```python
from build123d import *

# Parameters (mm, degrees)
SKETCH1_R                = 62.5
BOSS_EXTRUDE1_DEPTH      = 8
BOSS_EXTRUDE1_DEPTH_BACK = 8
SKETCH2_R                = 55
CUT_EXTRUDE1_DEPTH       = 5
SKETCH3_R                = 55
CUT_EXTRUDE2_DEPTH       = 5
SKETCH4_R                = 5
CUT_EXTRUDE3_DEPTH       = 12
SKETCH5_W                = 5
SKETCH5_H                = 25
CUT_EXTRUDE4_DEPTH       = 12
CIRPATTERN1_COUNT        = 4


with BuildPart() as part:
    # Sketch1 → Boss-Extrude1 (new body, two sides)
    with BuildSketch(Plane(origin=(0, 0, 0), x_dir=(1, 0, 0), z_dir=(0, 1, 0))) as boss_extrude1_sk:
        Circle(SKETCH1_R)
    extrude(amount=BOSS_EXTRUDE1_DEPTH)
    extrude(boss_extrude1_sk.sketch, amount=-BOSS_EXTRUDE1_DEPTH_BACK)

    # Sketch2 → Cut-Extrude1 (cut)
    with BuildSketch(Plane(origin=(0, 8, 0), x_dir=(1, 0, 0), z_dir=(0, 1, 0))):
        Circle(SKETCH2_R)
    extrude(amount=-CUT_EXTRUDE1_DEPTH, mode=Mode.SUBTRACT)

    # Sketch3 → Cut-Extrude2 (cut)
    with BuildSketch(Plane.XZ.offset(8)):
        Circle(SKETCH3_R)
    extrude(amount=-CUT_EXTRUDE2_DEPTH, mode=Mode.SUBTRACT)

    # Sketch4 → Cut-Extrude3 (cut, through all)
    with BuildSketch(Plane.XZ.offset(3)):
        Circle(SKETCH4_R)
    extrude(amount=-CUT_EXTRUDE3_DEPTH, mode=Mode.SUBTRACT)

    # Sketch5 → Cut-Extrude4 (cut, through all)
    with BuildSketch(Plane.XZ.offset(3)):
        with Locations((0, 40)):
            Rectangle(SKETCH5_W, SKETCH5_H)
    cut_extrude4 = extrude(amount=-CUT_EXTRUDE4_DEPTH, mode=Mode.SUBTRACT)

    # CirPattern1: Cut-Extrude4 ×4 about axis
    cirpattern1_axis = Axis((0, 0, 0), (0, 1, 0))
    for i in range(1, CIRPATTERN1_COUNT):
        add(cut_extrude4.rotate(cirpattern1_axis, i * 360 / CIRPATTERN1_COUNT), mode=Mode.SUBTRACT)


solid = part.part
```
Work out the finished part from the listing and answer in its coordinate system (mm). A direction names the side the tool comes from. Give positions to 0.01 mm unless a question says otherwise; leave off trailing zeros. Loops run counter-clockwise (first coordinate to the right, second up) from the corner with the lowest first, then second, coordinate; pieces in that order, holes last. Notation, with made-up numbers: (2, 47) -> (23, 47) arc R21 ccw to (23, 51) -> close; hole circle Ø4 at (-34, 39). An arc over 180 degrees is marked (long way). Use CSV: the item, a comma, the result in double quotes.
1. The part is cut by section D-D (z = 30). Write down the section's boundary in (x, y).
Found:
outline,"(-54.83, -8) -> (-46.1, -8) -> (-46.1, -3) -> (-2.5, -3) -> (-2.5, 3) -> (-46.1, 3) -> (-46.1, 8) -> (-54.83, 8) -> close; (2.5, -3) -> (46.1, -3) -> (46.1, -8) -> (54.83, -8) -> (54.83, 8) -> (46.1, 8) -> (46.1, 3) -> (2.5, 3) -> close"
2. Straight lines are drawn through the part: line 1 (Z direction, x = 0, y = 1.8); line 2 (Z direction, x = 0, y = 6.25); line 3 (Y direction, x = 4.5, z = 32.5). For each, find the intervals that lie inside material, in ascending order.
Found:
line 1,"-62.5 to -52.5, -27.5 to -5, 5 to 27.5, 52.5 to 62.5"
line 2,"-62.5 to -55, 55 to 62.5"
line 3,"-3 to 3"
3. The part is cut by section C-C (z = 0). Write down the section's boundary in (x, y).
Found:
outline,"(-62.5, -8) -> (-55, -8) -> (-55, -3) -> (-52.5, -3) -> (-52.5, 3) -> (-55, 3) -> (-55, 8) -> (-62.5, 8) -> close; (-27.5, -3) -> (-5, -3) -> (-5, 3) -> (-27.5, 3) -> close; (5, -3) -> (27.5, -3) -> (27.5, 3) -> (5, 3) -> close; (52.5, -3) -> (55, -3) -> (55, -8) -> (62.5, -8) -> (62.5, 8) -> (55, 8) -> (55, 3) -> (52.5, 3) -> close"
4. Flat-ended cylindrical pins translate along their axes: pin 1 Ø6 at (x, z) = (15.5, -46.5) entering from +Y; pin 2 Ø1.5 at (y, z) = (0, -0.5) entering from +X; pin 3 Ø3 at (x, y) = (-34.5, 0.5) entering from -Z; pin 4 Ø1.8 at (y, z) = (1, -35.5) entering from +X. Find the tip coordinate at first contact, or state that the pin passes through.
Found:
pin 1,"y = 3"
pin 2,"x = 62.5"
pin 3,"z = -53.08"
pin 4,"x = 52.05"
5. The part is cut by section A-A (x = 0). Write down the section's boundary in (y, z), then the cut area to 3 significant figures.
Found:
outline,"(-8, -62.5) -> (8, -62.5) -> (8, -55) -> (3, -55) -> (3, -52.5) -> (-3, -52.5) -> (-3, -55) -> (-8, -55) -> close; (-8, 55) -> (-3, 55) -> (-3, 52.5) -> (3, 52.5) -> (3, 55) -> (8, 55) -> (8, 62.5) -> (-8, 62.5) -> close; (-3, -27.5) -> (3, -27.5) -> (3, -5) -> (-3, -5) -> close; (-3, 5) -> (3, 5) -> (3, 27.5) -> (-3, 27.5) -> close"
area,"540 mm^2"
6. A tool of negligible diameter and unlimited length cuts with its end or side. For faces 4 (the cylindrical face through (-11.923, -5.535, -53.692)), 5 (the cylindrical face through (-11.923, 5.535, 53.692)), 6 (the flat face through (40, 0, -2.5)), from which of +Z, -Z, +X, -X, +Y, -Y can it reach the whole face along a straight path? Write none if from no direction.
Found:
face 4,"-Y"
face 5,"+Y"
face 6,"+Y, -Y"
7. The mould has two halves that part along X. Classify faces 1 (the flat face through (27.5, 0, 0)), 2 (the cylindrical face through (-62.44, 0.11, -2.75)), 3 (the flat face through (-0.3, 8, 55.3)): +X half, -X half, draft (parallel to the pull), parting line (faces both ways), or undercut.
Found:
face 1,"undercut"
face 2,"parting line"
face 3,"draft"
8. The part is cut by section B-B (y = 0). Write down the section's boundary in (x, z).
Found:
outline,"circle Ø125 at (0, 0); hole (-52.5, -2.5) -> (-27.5, -2.5) -> (-27.5, 2.5) -> (-52.5, 2.5) -> close; hole circle Ø10 at (0, 0); hole (-2.5, -52.5) -> (2.5, -52.5) -> (2.5, -27.5) -> (-2.5, -27.5) -> close; hole (-2.5, 27.5) -> (2.5, 27.5) -> (2.5, 52.5) -> (-2.5, 52.5) -> close; hole (27.5, -2.5) -> (52.5, -2.5) -> (52.5, 2.5) -> (27.5, 2.5) -> close"
